```python
from build123d import *

# Parameters (mm, degrees)
SKETCH_1_R          = 3.5
EXTRUDE_1_DEPTH     = 4.14
SKETCH_2_R          = 2
EXTRUDE_2_DEPTH     = 10
FILLET_1_R          = 0.5
CUT_EXTRUDE_1_DEPTH = 2


with BuildPart() as part:
    # 草图1 → 凸台-拉伸1 (new body)
    with BuildSketch(Plane(origin=(0, 0, 0), x_dir=(1, 0, 0), z_dir=(0, 1, 0))):
        with Locations(Location((0, 0, 0), (0, 0, 270))):
            Circle(SKETCH_1_R)
    extrude(amount=EXTRUDE_1_DEPTH)

    # 草图2 → 凸台-拉伸2 (add)
    with BuildSketch(Plane(origin=(0, 4.14, 0), x_dir=(1, 0, 0), z_dir=(0, 1, 0))):
        with Locations(Location((0, 0, 0), (0, 0, 270))):
            Circle(SKETCH_2_R)
    extrude(amount=EXTRUDE_2_DEPTH)

    # 圆角1
    fillet_1_edges = [part.edges().sort_by_distance(p)[0] for p in [
        (0, 0, -3.5),
    ]]
    fillet(fillet_1_edges, radius=FILLET_1_R)

    # 草图3 → 切除-拉伸1 (cut)
    with BuildSketch(Plane.XZ):
        Polygon((1.698287208, 2.056072434), (-0.931467356, 2.498796082), (-2.629754564, 0.442723648), (-1.698287208, -2.056072434), (0.931467356, -2.498796082), (2.629754564, -0.442723648), align=None)
    extrude(amount=-CUT_EXTRUDE_1_DEPTH, mode=Mode.SUBTRACT)


solid = part.part
```
Design review of the part built by this model. Coordinates are the model's own, in mm. A direction names the side the tool comes from. Round coordinates to 2 decimals unless told otherwise and drop trailing zeros. Write each loop counter-clockwise with the first axis right and the second up, starting at its lowest first coordinate (ties: lowest second). Pieces come first, ordered by that corner, then holes. Notation, with made-up numbers: (-1.75, 40) -> (3.25, 40) arc R21 ccw to (3.25, 56) -> close; hole circle Ø9 at (35, -38). An arc over 180 degrees is marked (long way). Answer in a Markdown table with one row per item.
Q1. Take a section at A-A, the plane z = 0. State the section outline as (x, y) points, then the cut area to 3 significant figures.
The answers:
| item | result |
|---|---|
| outline | (-3.5, 0.5) arc R0.5 ccw to (-3, 0) -> (-2.46, 0) -> (-2.46, 2) -> (2.46, 2) -> (2.46, 0) -> (3, 0) arc R0.5 ccw to (3.5, 0.5) -> (3.5, 4.14) -> (2, 4.14) -> (2, 14.14) -> (-2, 14.14) -> (-2, 4.14) -> (-3.5, 4.14) -> close |
| area | 59.0 mm² |
Q2. For faces 5 (the face through (-2, 4.14, 2)), 6 (the face through (-2, 0, 2)), 7 (the face through (-2.17, 0.99, -0.79)), list the 3-axis set-ups (+Z, -Z, +X, -X, +Y, -Y) from which the entire face can be reached by the end or side of a thin tool; tool diameter is ignored.
The answers:
| item | result |
|---|---|
| face 5 | +Y |
| face 6 | +Z, -Z, +X, -X, -Y |
| face 7 | -Y |
Q3. Draft analysis for pull direction Z (two halves, no side actions). For faces 1 (the face through (0, 2, 0)), 2 (the face through (-2, 9, 0)), 3 (the face through (2.17, 0.99, 0.79)), 4 (the face through (0, 14.14, 0)), state which applies: +Z half, -Z half, draft (parallel to the pull), parting line (faces both ways), or undercut.
The answers:
| item | result |
|---|---|
| face 1 | undercut |
| face 2 | parting line |
| face 3 | undercut |
| face 4 | draft |
Q4. To check wall thickness, follow L1, parallel to Y at x = 0, z = 1.5; L2, parallel to Y at x = -2.5, z = -1; L3, parallel to Z at x = 0.5, y = 8. State the ranges of each line that lie inside material, in increasing order. Write a range as [from, to].
The answers:
| item | result |
|---|---|
| L1 | [2, 14.14] |
| L2 | [0, 4.14] |
| L3 | [-1.94, 1.94] |
Q5. Take a section at B-B, the plane y = 7.5. State the section outline as (x, z) points, then the cut area to 3 significant figures.
The answers:
| item | result |
|---|---|
| outline | circle Ø4 at (0, 0) |
| area | 12.6 mm² |
Q6. Take a section at C-C, the plane x = 0. State the section outline as (y, z) points, then the cut area to 3 significant figures.
The answers:
| item | result |
|---|---|
| outline | (0, -3) arc R0.5 ccw to (0.5, -3.5) -> (4.14, -3.5) -> (4.14, -2) -> (14.14, -2) -> (14.14, 2) -> (4.14, 2) -> (4.14, 3.5) -> (0.5, 3.5) arc R0.5 ccw to (0, 3) -> (0, 2.34) -> (2, 2.34) -> (2, -2.34) -> (0, -2.34) -> close |
| area | 59.5 mm² |
Q7. Clearance check with flat-ended pins moving along their axes: pin 1 Ø1.5 at (x, y) = (1.5, 10.5) entering from +Z; pin 2 Ø1.5 at (y, z) = (9.5, 1) entering from +X; pin 3 Ø3 at (x, y) = (-2, 4.5) entering from +Z. State where each tip first meets the part, or that it passes through.
The answers:
| item | result |
|---|---|
| pin 1 | z = 1.85 |
| pin 2 | x = 1.98 |
| pin 3 | z = 3.46 |
